Part model, mm, in its own coordinate system. Face numbers are marked on the shaded views. A direction names the side the tool comes from. Round coordinates to 2 decimals unless told otherwise and drop trailing zeros. Loops run counter-clockwise (first coordinate to the right, second up) from the corner with the lowest first, then second, coordinate; pieces in that order, holes last. Notation, with made-up numbers: (-1.75, 29) -> (22.25, 29) arc R18 ccw to (22.25, 63) -> close; hole circle Ø1 at (-26, -37.5). An arc over 180 degrees is marked (long way). Use a Markdown table: item, result. Add a question column.
Item 1: Flat gauge pins, fed straight in: pin 1 (23.5 mm diameter, centred on y = 60.5, z = -43.5, fed in from +X); pin 2 (10 mm diameter, centred on x = 55.5, z = -55, fed in from +Y); pin 3 (23.5 mm diameter, centred on y = 61, z = -42, fed in from -X). Where does each tip first touch, or does it go through?
Item 2: Cut at A-A, the plane x = -77. List the corners of the cut face in (y, z), plus the area to 3 significant figures.
Item 3: Probe line 1 (Z direction, x = -40, y = 3); line 2 (Y direction, x = 88, z = -41); line 3 (X direction, y = 43, z = -72.5). List the from-to ranges inside material, lowest first. Write a range as [from, to].
Item 4: Which spindle directions (+Z, -Z, +X, -X, +Y, -Y) get a long thin tool onto all of the face, cutting with end or side? Do the marked faces 5, 6, 7 and 8. Say none if no direction does.
Item 5: Cut at D-D, the plane z = -55. List the corners of the cut face in (x, y), plus the area to 3 significant figures.
Item 6: Two-plate mould, pull along X, no slides. Class the marked faces 1, 2, 3 and 4: pulls with the +X half, pulls with the -X half, needs draft (parallel to the pull), parting line crosses it, or undercut.
Item 7: Cut at C-C, the plane y = 28. List the corners of the cut face in (x, z).
Item 8: Cut at B-B, the plane y = 82. State how many separate pieces and enclosed holes the cut face has, plus the area to 3 significant figures.
```python
from build123d import *

# Parameters (mm, degrees)
BOSS_EXTRUDE1_DEPTH      = 82
SKETCH5_R                = 11
CUT_EXTRUDE1_DEPTH       = 13
CUT_EXTRUDE2_REACH       = 4
SKETCH6_R                = 10
FILLET1_R                = 0.3
CUT_EXTRUDE4_REACH       = 22
SKETCH8_R                = 28
CUT_EXTRUDE5_REACH       = 96
FILLET3_R                = 25
FILLET7_R                = 10
CUT_EXTRUDE7_DEPTH       = 10
M4_CLEARANCE_HOLE2_D     = 4.5
M4_CLEARANCE_HOLE2_DEPTH = 10
M4_CLEARANCE_HOLE2_TIP   = 1.351936393
M4_CLEARANCE_HOLE3_D     = 4.5
M4_CLEARANCE_HOLE3_DEPTH = 20


with BuildPart() as part:
    # Sketch1 → Boss-Extrude1 (new body)
    with BuildSketch(Plane.XY):
        Polygon((0, 0), (-74, 0), (-94, 0), (-94, 98), (-74, 98), (-74, 20), (-15, 20), (-15, 74), (0, 74), align=None)
    extrude(amount=-BOSS_EXTRUDE1_DEPTH)

    # Sketch5 → Cut-Extrude1 (cut)
    with BuildSketch(Plane.ZY.offset(15)):
        with Locations((-41, 58)):
            Circle(SKETCH5_R)
    extrude(amount=-CUT_EXTRUDE1_DEPTH, mode=Mode.SUBTRACT)

    # Sketch6 → Cut-Extrude2 (cut, up to next)
    with BuildSketch(Plane.ZY.offset(2), mode=Mode.PRIVATE) as cut_extrude2_sk1:
        with Locations((-41, 58)):
            Circle(SKETCH6_R)
    cut_extrude2_tool1 = extrude(cut_extrude2_sk1.sketch, amount=-CUT_EXTRUDE2_REACH, mode=Mode.PRIVATE) & part.part
    add(cut_extrude2_tool1.solids().sort_by_distance((-2, 58, -41))[0], mode=Mode.SUBTRACT)

    # Fillet1
    fillet1_edges = [part.edges().sort_by_distance(p)[0] for p in [
        (-2, 58, -52),
    ]]
    fillet(fillet1_edges, radius=FILLET1_R)

    # Sketch8 → Cut-Extrude4 (cut, up to next)
    with BuildSketch(Plane(origin=(-74, 0, 0), x_dir=(0, 0, -1), z_dir=(1, 0, 0)), mode=Mode.PRIVATE) as cut_extrude4_sk1:
        with Locations((41, 58)):
            Circle(SKETCH8_R)
    cut_extrude4_tool1 = extrude(cut_extrude4_sk1.sketch, amount=-CUT_EXTRUDE4_REACH, mode=Mode.PRIVATE) & part.part
    add(cut_extrude4_tool1.solids().sort_by_distance((-74, 58, -41))[0], mode=Mode.SUBTRACT)

    # Sketch10 → Cut-Extrude5 (cut, up to next)
    with BuildSketch(Plane(origin=(0, 0, 0), x_dir=(0, 0, -1), z_dir=(1, 0, 0)), mode=Mode.PRIVATE) as cut_extrude5_sk1:
        with BuildLine():
            Line((0, 74), (0, 20))
            Line((0, 20), (25, 20))
            Line((25, 20), (25, 58))
            ThreePointArc((25, 58), (29.686291501, 69.313708499), (41, 74))
            Line((41, 74), (0, 74))
        make_face()
    cut_extrude5_tool1 = extrude(cut_extrude5_sk1.sketch, amount=-CUT_EXTRUDE5_REACH, mode=Mode.PRIVATE) & part.part
    add(cut_extrude5_tool1.solids().sort_by_distance((0, 47.916044, -13.128546))[0], mode=Mode.SUBTRACT)
    # Sketch10 → Cut-Extrude5 (cut, up to next)
    with BuildSketch(Plane(origin=(0, 0, 0), x_dir=(0, 0, -1), z_dir=(1, 0, 0)), mode=Mode.PRIVATE) as cut_extrude5_sk2:
        with BuildLine():
            Line((82, 74), (41, 74))
            ThreePointArc((41, 74), (52.313708499, 69.313708499), (57, 58))
            Line((57, 58), (57, 20))
            Line((57, 20), (82, 20))
            Line((82, 20), (82, 74))
        make_face()
    cut_extrude5_tool2 = extrude(cut_extrude5_sk2.sketch, amount=-CUT_EXTRUDE5_REACH, mode=Mode.PRIVATE) & part.part
    add(cut_extrude5_tool2.solids().sort_by_distance((0, 47.916044, -68.871454))[0], mode=Mode.SUBTRACT)

    # Fillet3
    fillet3_edges = [part.edges().sort_by_distance(p)[0] for p in [
        (-84, 98, 0),
        (-84, 98, -82),
    ]]
    fillet(fillet3_edges, radius=FILLET3_R)

    # Fillet7
    fillet7_edges = [part.edges().sort_by_distance(p)[0] for p in [
        (-7.5, 20, -57),
        (-7.5, 20, -25),
    ]]
    fillet(fillet7_edges, radius=FILLET7_R)

    # Sketch16 → Cut-Extrude7 (cut)
    with BuildSketch(Plane.XZ):
        with BuildLine():
            Line((0, -9.457), (0, -14.457))
            ThreePointArc((0, -14.457), (-26.543, -41), (0, -67.543))
            Line((0, -67.543), (0, -72.543))
            ThreePointArc((0, -72.543), (-31.543, -41), (0, -9.457))
        make_face()
    extrude(amount=-CUT_EXTRUDE7_DEPTH, mode=Mode.SUBTRACT)

    # M4 Clearance Hole2
    with Locations(Plane(origin=(0, 0, 0), x_dir=(-1, 0, 0), z_dir=(0, -1, 0))):
        with Locations((40, 9.457), (40, 72.543)):
            Hole(M4_CLEARANCE_HOLE2_D / 2, depth=M4_CLEARANCE_HOLE2_DEPTH)
            with Locations((0, 0, -(M4_CLEARANCE_HOLE2_DEPTH + M4_CLEARANCE_HOLE2_TIP / 2))):  # 118° drill point
                Cone(0, M4_CLEARANCE_HOLE2_D / 2, M4_CLEARANCE_HOLE2_TIP, mode=Mode.SUBTRACT)

    # M4 Clearance Hole3
    with Locations(Plane.ZY.offset(94)):
        with Locations((-70, 28), (-12, 28), (-12, 82), (-70, 82)):
            Hole(M4_CLEARANCE_HOLE3_D / 2, depth=M4_CLEARANCE_HOLE3_DEPTH)

    # Mirror1: part across plane


with BuildPart() as part_1:
    add(part.part)
    add(part.part.mirror(Plane(origin=(0, 74, -82), x_dir=(0, 0, 1), z_dir=(1, 0, 0))))


solid = part_1.part
```
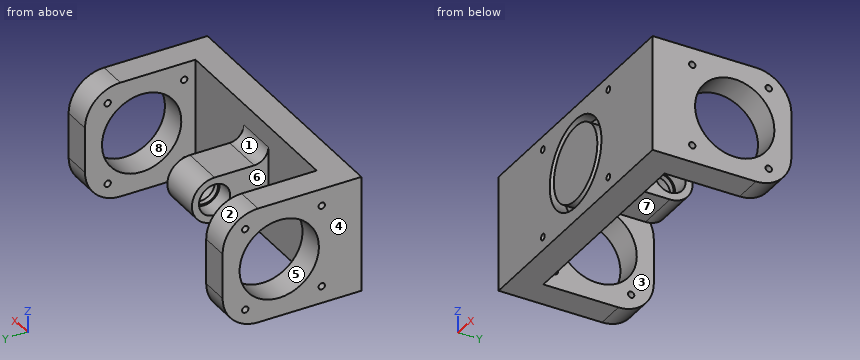
A:
| question | item | result |
|---|---|---|
| 1 | pin 1 | stops at x = 15 |
| 1 | pin 2 | stops at y = 20 |
| 1 | pin 3 | stops at x = -15 |
| 2 | outline | (0, -82) -> (73, -82) arc R25 ccw to (98, -57) -> (98, -25) arc R25 ccw to (73, 0) -> (0, 0) -> close; hole circle Ø4.5 at (28, -70); hole circle Ø4.5 at (28, -12); hole circle Ø56 at (58, -41); hole circle Ø4.5 at (82, -70); hole circle Ø4.5 at (82, -12) |
| 2 | area | 5,240 mm^2 |
| 3 | line 1 | z = [-82, -74.79], [-70.29, -11.71], [-7.21, 0] |
| 3 | line 2 | y = [0, 30], [86, 98] |
| 3 | line 3 | x = [-94, -74], [74, 94] |
| 4 | face 5 | -X |
| 4 | face 6 | +Z, -Z, +Y |
| 4 | face 7 | -Z, +Y |
| 4 | face 8 | +X |
| 5 | outline | (-94, 0) -> (-28.27, 0) -> (-28.27, 10) -> (-22.55, 10) -> (-22.55, 0) -> (22.55, 0) -> (22.55, 10) -> (28.27, 10) -> (28.27, 0) -> (94, 0) -> (94, 33.75) -> (74, 33.75) -> (74, 20) -> (15, 20) -> (15, 65.75) -> (-15, 65.75) -> (-15, 20) -> (-74, 20) -> (-74, 33.75) -> (-94, 33.75) -> close; (-94, 82.25) -> (-74, 82.25) -> (-74, 98) -> (-94, 98) -> close; (74, 82.25) -> (94, 82.25) -> (94, 98) -> (74, 98) -> close |
| 5 | area | 6,200 mm^2 |
| 6 | face 1 | undercut |
| 6 | face 2 | needs draft |
| 6 | face 3 | undercut |
| 6 | face 4 | pulls with the -X half |
| 7 | outline | (-94, -82) -> (-74, -82) -> (-74, -72.25) -> (-94, -72.25) -> close; (-94, -67.75) -> (-74, -67.75) -> (-74, -14.25) -> (-94, -14.25) -> close; (-94, -9.75) -> (-74, -9.75) -> (-74, 0) -> (-94, 0) -> close; (-15, -57.2) -> (15, -57.2) -> (15, -24.8) -> (-15, -24.8) -> close; (74, -82) -> (94, -82) -> (94, -72.25) -> (74, -72.25) -> close; (74, -67.75) -> (94, -67.75) -> (94, -14.25) -> (74, -14.25) -> close; (74, -9.75) -> (94, -9.75) -> (94, 0) -> (74, 0) -> close |
| 8 | separate pieces | 8 |
| 8 | enclosed holes | 0 |
| 8 | area | 1,630 mm^2 |
